The figure shows three views and two pictorial views of one solid part (mm, origin at its lowest corner). Answer the questions. A direction names the side the tool comes from. Round coordinates to 2 decimals unless told otherwise and drop trailing zeros. Order: outer loops, then holes, each group sorted by start corner. A loop starts at its lowest first (then second) coordinate and runs counter-clockwise, first axis right, second up. Notation, with made-up numbers: (1.25, -20.75) - (23.25, -20.75) arc R24 cw to (23.25, -5.75) - close; hole circle Ø10 at (-8.75, -3). An arc over 180 degrees is marked (long way). One line per item, written item: value. Start each with the question number.
1. Section B-B, the plane x = 9 is taken. Give the vertices of the cut face in (y, z), then the cut area to 3 significant figures.
2. A straight line is drawn through the part: line 1 (X direction, y = 22.75, z = 49.5). Find the intervals that lie inside material, in ascending order.
3. A tool of negligible diameter and unlimited length cuts with its end or side. For the marked faces 1, 2 and 3, from which of +Z, -Z, +X, -X, +Y, -Y can it reach the whole face along a straight path? Write none if from no direction.
4. Section A-A, the plane z = 22 is taken. Give the vertices of the cut face in (x, y), then the cut area to 3 significant figures.
5. Flat-ended cylindrical pins translate along their axes: P1, Ø8, axis at y = 14.5, z = 69, coming from the -X side; P2, Ø1.5, axis at x = 9.5, y = 25, coming from the +Z side; P3, Ø1, axis at x = 71, y = 19.5, coming from the -Z side. Find the tip coordinate at first contact, or state that the pin passes through.
6. Section C-C, the plane y = 25.75 is taken. Give the vertices of the cut face in (x, z), then the cut area to 3 significant figures.
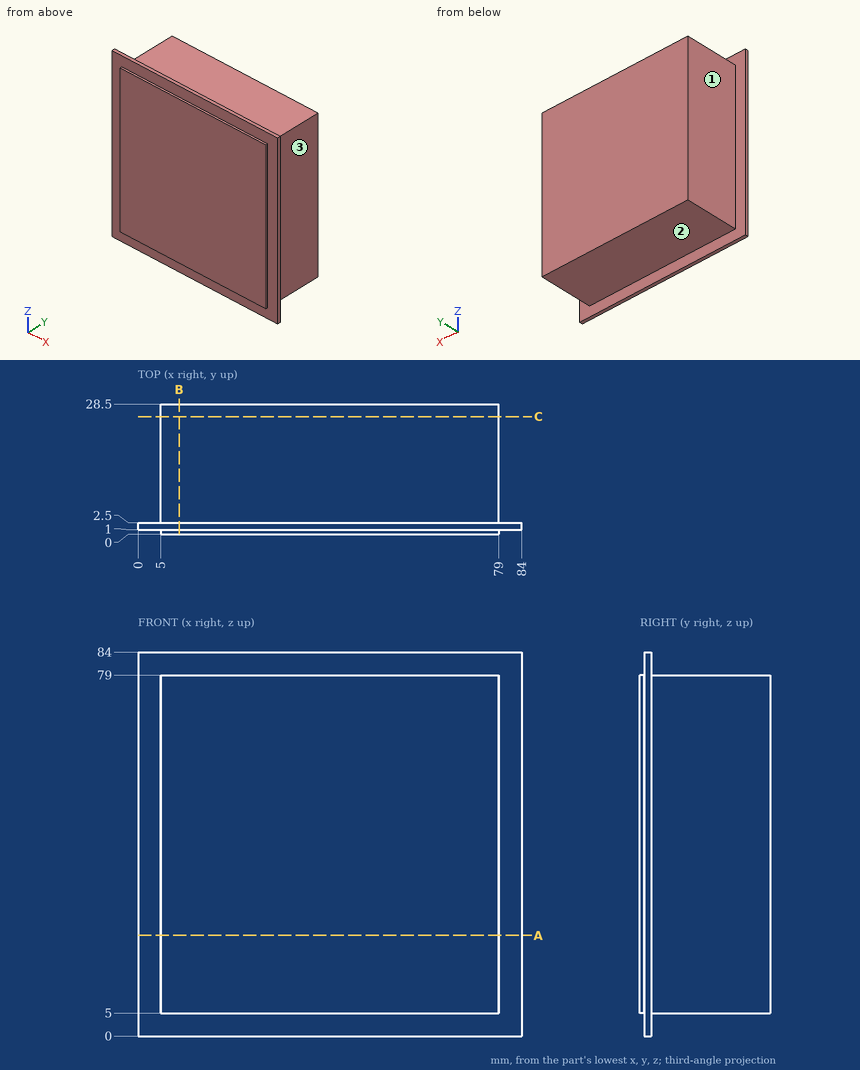
Answer list:
1. outline: (0, 5) - (1, 5) - (1, 0) - (2.5, 0) - (2.5, 5) - (28.5, 5) - (28.5, 79) - (2.5, 79) - (2.5, 84) - (1, 84) - (1, 79) - (0, 79) - close
1. area: 2,120 mm²
2. line 1: x = 5 to 79
3. face 1: +Z, -Z, -X, +Y
3. face 2: -Z, +X, -X, +Y
3. face 3: +Z, -Z, +X, +Y
4. outline: (0, 1) - (5, 1) - (5, 0) - (79, 0) - (79, 1) - (84, 1) - (84, 2.5) - (79, 2.5) - (79, 28.5) - (5, 28.5) - (5, 2.5) - (0, 2.5) - close
4. area: 2,120 mm²
5. P1: stops at x = 5
5. P2: stops at z = 79
5. P3: stops at z = 5
6. outline: (5, 5) - (79, 5) - (79, 79) - (5, 79) - close
6. area: 5,480 mm²
